Verification items for the finished model (mm, model axes). A direction names the side the tool comes from. Coordinates: 2 decimals unless noted, no trailing zeros. Write each loop counter-clockwise with the first axis right and the second up, starting at its lowest first coordinate (ties: lowest second). Pieces come first, ordered by that corner, then holes. Notation, with made-up numbers: (87.5, 73) -> (124.5, 73) arc R15 ccw to (124.5, 101) -> close; hole circle Ø7 at (-19, 44.5). An arc over 180 degrees is marked (long way). Answer in a Markdown table with one row per item.
```python
from build123d import *

# Parameters (mm, degrees)
SKETCH_1_R          = 35
SKETCH_1_R_2        = 2
EXTRUDE_1_DEPTH     = 2.5
SKETCH_2_R          = 5
EXTRUDE_2_DEPTH     = 5
EXTRUDE_3_DEPTH     = 2
EXTRUDE_START       = -2
EXTRUDE_4_DEPTH     = 2
SKETCH_6_R          = 2.5
CUT_EXTRUDE_1_DEPTH = 51.062460986


with BuildPart() as part:
    # 草图1 → 凸台-拉伸1 (new body)
    with BuildSketch(Plane.XY):
        Circle(SKETCH_1_R)
        with Locations((17.25, 0)):
            Circle(SKETCH_1_R_2, mode=Mode.SUBTRACT)
        with Locations((8.625, -14.938938215)):
            Circle(SKETCH_1_R_2, mode=Mode.SUBTRACT)
        with Locations((-8.625, -14.938938215)):
            Circle(SKETCH_1_R_2, mode=Mode.SUBTRACT)
        with Locations((-17.25, 0)):
            Circle(SKETCH_1_R_2, mode=Mode.SUBTRACT)
        with Locations((-8.625, 14.938938215)):
            Circle(SKETCH_1_R_2, mode=Mode.SUBTRACT)
        with Locations((8.625, 14.938938215)):
            Circle(SKETCH_1_R_2, mode=Mode.SUBTRACT)
    extrude(amount=EXTRUDE_1_DEPTH)

    # 草图2 → 凸台-拉伸2 (add)
    with BuildSketch(Plane(origin=(0, 0, 0), x_dir=(-1, 0, 0), z_dir=(0, 0, -1))):
        with Locations(Location((0, 0, 0), (0, 0, 180))):
            Circle(SKETCH_2_R)
    extrude(amount=EXTRUDE_2_DEPTH)

    # 草图3 → 凸台-拉伸3 (add)
    with BuildSketch(Plane(origin=(0, 0, -5), x_dir=(-1, 0, 0), z_dir=(0, 0, -1))):
        with BuildLine():
            Line((1.910748146, -3.264034868), (-23.979362284, -18.419963804))
            ThreePointArc((-23.979362284, -18.419963804), (-29.154145298, -17.066677082), (-27.800858576, -11.891894068))
            Line((-27.800858576, -11.891894068), (-1.910748146, 3.264034868))
            ThreePointArc((-1.910748146, 3.264034868), (3.264034868, 1.910748146), (1.910748146, -3.264034868))
        make_face()
    extrude(amount=-EXTRUDE_3_DEPTH)

    # 草图5 → 凸台-拉伸4 (add)
    with BuildSketch(Plane(origin=(0, 0, -5), x_dir=(-1, 0, 0), z_dir=(0, 0, -1)).offset(EXTRUDE_START)):
        with BuildLine():
            Line((23.995619313, 18.39219274), (0.959625284, 4.907047923))
            ThreePointArc((0.959625284, 4.907047923), (4.315018405, 2.525988156), (4.748607518, -1.565479685))
            Line((4.748607518, -1.565479685), (27.784601547, 11.919665132))
            ThreePointArc((27.784601547, 11.919665132), (29.126374234, 17.050420053), (23.995619313, 18.39219274))
        make_face()
    extrude(amount=EXTRUDE_4_DEPTH)

    # 草图6 → 切除-拉伸1 (cut, through all)
    with BuildSketch(Plane(origin=(0, 0, -5), x_dir=(-1, 0, 0), z_dir=(0, 0, -1))):
        with Locations((-25.89011043, -15.155928936)):
            Circle(SKETCH_6_R)
        with Locations((25.89011043, 15.155928936)):
            Circle(SKETCH_6_R)
    extrude(amount=-CUT_EXTRUDE_1_DEPTH, mode=Mode.SUBTRACT)


solid = part.part
```
1. Material ranges on probe 1 along Z at (x, y) = (17.5, -7.5); probe 2 along X at (y, z) = (15, 2.25); probe 3 along Z at (x, y) = (-1.5, -26), recorded low to high. Write a range as from..to.
Findings below:
| item | result |
|---|---|
| probe 1 | z = -5..-3, 0..2.5 |
| probe 2 | x = -31.62..-28.39, -23.39..-10.62, -6.63..6.63, 10.62..31.62 |
| probe 3 | z = 0..2.5 |
2. Sectioned sample at C-C, the plane x = -17.25. Record the cut outline in (y, z).
Findings below:
| item | result |
|---|---|
| outline | (-30.45, 0) -> (-2, 0) -> (-2, 2.5) -> (-30.45, 2.5) -> close; (2, 0) -> (30.45, 0) -> (30.45, 2.5) -> (2, 2.5) -> close; (5.75, -5) -> (14.44, -5) -> (14.44, -3) -> (5.75, -3) -> close |
3. Access from +Z, -Z, +X, -X, +Y, -Y to the whole of each face (thin tool, end or side, straight path). Record for faces 1 (the face through (-18.837, -1.217, 1.232)), 2 (the face through (4.77, -1.5, -1.91)).
Findings below:
| item | result |
|---|---|
| face 1 | +Z, -Z |
| face 2 | none |
4. Sectioned sample at A-A, the plane x = 14. Record the cut outline in (y, z), and give its area (3 significant figures).
Findings below:
| item | result |
|---|---|
| outline | (-32.08, 0) -> (32.08, 0) -> (32.08, 2.5) -> (-32.08, 2.5) -> close; (-12.58, -5) -> (-3.81, -5) -> (-3.81, -3) -> (-12.58, -3) -> close |
| area | 178 mm² |
5. Go/stop test with flat-tipped pins: pin 1 (6.5 mm diameter, centred on x = 17.25, y = 0, fed in from +Z); pin 2 (2 mm diameter, centred on y = -7, z = 0.5, fed in from -X); pin 3 (2 mm diameter, centred on x = -4, z = -1.5, fed in from -Y); pin 4 (2 mm diameter, centred on y = -9.5, z = -3.5, fed in from -X). Record where each tip stops, or that it passes through.
Findings below:
| item | result |
|---|---|
| pin 1 | stops at z = 2.5 |
| pin 2 | stops at x = -34.48 |
| pin 3 | stops at y = -4 |
| pin 4 | stops at x = 7.03 |
6. Sectioned sample at D-D, the plane y = 0. Record the cut outline in (x, z), and give its area (3 significant figures).
Findings below:
| item | result |
|---|---|
| outline | (-35, 0) -> (-19.25, 0) -> (-19.25, 2.5) -> (-35, 2.5) -> close; (-15.25, 0) -> (-5, 0) -> (-5, -3) -> (-7.42, -3) -> (-7.42, -5) -> (7.49, -5) -> (7.49, -3) -> (5, -3) -> (5, 0) -> (15.25, 0) -> (15.25, 2.5) -> (-15.25, 2.5) -> close; (19.25, 0) -> (35, 0) -> (35, 2.5) -> (19.25, 2.5) -> close |
| area | 215 mm² |
7. Release check for a two-part mould opening along X. For faces 3 (the face through (7, 0, 0)), 4 (the face through (-28, -21, 1)), 5 (the face through (15.663, -1.217, 1.232)), 6 (the face through (-16.105, 5.083, -3.986)) record: released by +X, released by -X, zero draft, split by the parting line, or undercut.
Findings below:
| item | result |
|---|---|
| face 3 | zero draft |
| face 4 | split by the parting line |
| face 5 | undercut |
| face 6 | released by -X |
8. Sectioned sample at B-B, the plane y = 14. Record the cut outline in (x, z), and give its area (3 significant figures).
Findings below:
| item | result |
|---|---|
| outline | (-32.08, 0) -> (-28.11, 0) -> (-28.11, 2.5) -> (-32.08, 2.5) -> close; (-29.46, -5) -> (-28.11, -5) -> (-28.11, -3) -> (-29.46, -3) -> close; (-23.67, -5) -> (-16.49, -5) -> (-16.49, -3) -> (-23.67, -3) -> close; (-23.67, 0) -> (-10.39, 0) -> (-10.39, 2.5) -> (-23.67, 2.5) -> close; (-6.86, 0) -> (6.86, 0) -> (6.86, 2.5) -> (-6.86, 2.5) -> close; (10.39, 0) -> (32.08, 0) -> (32.08, 2.5) -> (10.39, 2.5) -> close |
| area | 149 mm² |
